Work out the finished part from the listing and answer in its coordinate system (mm). A direction names the side the tool comes from. Coordinates: 2 decimals unless noted, no trailing zeros. Order: outer loops, then holes, each group sorted by start corner. A loop starts at its lowest first (then second) coordinate and runs counter-clockwise, first axis right, second up. Notation, with made-up numbers: M -28.75,-7 L -11.75,-7 A28 cw -11.75,29 Z; hole C 61.5,34.5 d1. An arc over 180 degrees is marked long. Use a Markdown table: item, result.
from build123d import *

# Parameters (mm, degrees)
SKETCH1_W           = 88.9
SKETCH1_H           = 50.8
BOSS_EXTRUDE1_DEPTH = 12.7
SKETCH2_R           = 3.429
SKETCH2_R_2         = 2.286
CUT_EXTRUDE1_DEPTH  = 4.572
SKETCH3_R           = 2.286
CUT_EXTRUDE2_DEPTH  = 53.74706153
LPATTERN1_COUNT     = 2
LPATTERN1_PITCH     = 25.4
CUT_EXTRUDE3_DEPTH  = 69.685751798
SKETCH5_R           = 0.7874
CUT_EXTRUDE4_DEPTH  = 53.74706153
SKETCH6_R           = 2.286
CUT_EXTRUDE5_DEPTH  = 53.74706153


with BuildPart() as part:
    # Sketch1 → Boss-Extrude1 (new body)
    with BuildSketch(Plane(origin=(0, 0, 0), x_dir=(1, 0, 0), z_dir=(0, 1, 0))):
        Rectangle(SKETCH1_W, SKETCH1_H)
    extrude(amount=BOSS_EXTRUDE1_DEPTH)

    # Sketch2 → Cut-Extrude1 (cut)
    # profile 1 of 5: a face of its own
    with BuildSketch(Plane(origin=(0, 12.7, 0), x_dir=(1, 0, 0), z_dir=(0, 1, 0))):
        with Locations(Location((-34.29, 12.7, 0), (0, 0, 270))):
            Circle(SKETCH2_R)
        with Locations(Location((-34.29, 12.7, 0), (0, 0, 270))):
            Circle(SKETCH2_R_2, mode=Mode.SUBTRACT)
    # profile 2 of 5: a face of its own
    with BuildSketch(Plane(origin=(0, 12.7, 0), x_dir=(1, 0, 0), z_dir=(0, 1, 0))):
        with Locations(Location((-19.05, 12.7, 0), (0, 0, 270))):
            Circle(SKETCH2_R)
        with Locations(Location((-19.05, 12.7, 0), (0, 0, 270))):
            Circle(SKETCH2_R_2, mode=Mode.SUBTRACT)
    # profile 3 of 5: a face of its own
    with BuildSketch(Plane(origin=(0, 12.7, 0), x_dir=(1, 0, 0), z_dir=(0, 1, 0))):
        with Locations(Location((0, 12.7, 0), (0, 0, 270))):
            Circle(SKETCH2_R)
        with Locations(Location((0, 12.7, 0), (0, 0, 270))):
            Circle(SKETCH2_R_2, mode=Mode.SUBTRACT)
    # profile 4 of 5: a face of its own
    with BuildSketch(Plane(origin=(0, 12.7, 0), x_dir=(1, 0, 0), z_dir=(0, 1, 0))):
        with Locations(Location((19.05, 12.7, 0), (0, 0, 270))):
            Circle(SKETCH2_R)
        with Locations(Location((19.05, 12.7, 0), (0, 0, 270))):
            Circle(SKETCH2_R_2, mode=Mode.SUBTRACT)
    # profile 5 of 5: a face of its own
    with BuildSketch(Plane(origin=(0, 12.7, 0), x_dir=(1, 0, 0), z_dir=(0, 1, 0))):
        with Locations(Location((34.29, 12.7, 0), (0, 0, 270))):
            Circle(SKETCH2_R)
        with Locations(Location((34.29, 12.7, 0), (0, 0, 270))):
            Circle(SKETCH2_R_2, mode=Mode.SUBTRACT)
    cut_extrude1 = extrude(amount=-CUT_EXTRUDE1_DEPTH, mode=Mode.SUBTRACT)

    # Sketch3 → Cut-Extrude2 (cut, through all)
    with BuildSketch(Plane(origin=(0, 12.7, 0), x_dir=(1, 0, 0), z_dir=(0, 1, 0))):
        with Locations(Location((-34.29, 12.7, 0), (0, 0, 270))):
            Circle(SKETCH3_R)
        with Locations(Location((-19.05, 12.7, 0), (0, 0, 270))):
            Circle(SKETCH3_R)
        with Locations(Location((0, 12.7, 0), (0, 0, 270))):
            Circle(SKETCH3_R)
        with Locations(Location((19.05, 12.7, 0), (0, 0, 270))):
            Circle(SKETCH3_R)
        with Locations(Location((34.29, 12.7, 0), (0, 0, 270))):
            Circle(SKETCH3_R)
    extrude(amount=-CUT_EXTRUDE2_DEPTH, mode=Mode.SUBTRACT)

    # LPattern1: Cut-Extrude1 ×2
    with Locations(*[(0, 0, i * LPATTERN1_PITCH) for i in range(1, LPATTERN1_COUNT)]):
        add(cut_extrude1, mode=Mode.SUBTRACT)

    # Sketch4 → Cut-Extrude3 (cut, through all)
    with BuildSketch(Plane.XY.offset(25.4)):
        with BuildLine():
            Line((-28.702, 0), (-22.098, 0))
            ThreePointArc((-22.098, 0), (-25.4, 3.302), (-28.702, 0))
        make_face()
        with BuildLine():
            Line((-14.224, 0), (-4.572, 0))
            ThreePointArc((-4.572, 0), (-9.398, 4.826), (-14.224, 0))
        make_face()
        with BuildLine():
            Line((4.572, 0), (14.224, 0))
            ThreePointArc((14.224, 0), (9.398, 4.826), (4.572, 0))
        make_face()
        with BuildLine():
            Line((22.098, 0), (28.702, 0))
            ThreePointArc((28.702, 0), (25.4, 3.302), (22.098, 0))
        make_face()
    extrude(amount=-CUT_EXTRUDE3_DEPTH, mode=Mode.SUBTRACT)

    # Sketch5 → Cut-Extrude4 (cut, through all)
    with BuildSketch(Plane(origin=(0, 12.7, 0), x_dir=(1, 0, 0), z_dir=(0, 1, 0))):
        with Locations(Location((0, 0, 0), (0, 0, 270))):
            Circle(SKETCH5_R)
    extrude(amount=-CUT_EXTRUDE4_DEPTH, mode=Mode.SUBTRACT)

    # Sketch6 → Cut-Extrude5 (cut, through all)
    with BuildSketch(Plane(origin=(0, 12.7, 0), x_dir=(1, 0, 0), z_dir=(0, 1, 0))):
        with Locations(Location((-34.29, -12.7, 0), (0, 0, 270))):
            Circle(SKETCH6_R)
        with Locations(Location((-19.05, -12.7, 0), (0, 0, 270))):
            Circle(SKETCH6_R)
        with Locations(Location((0, -12.7, 0), (0, 0, 270))):
            Circle(SKETCH6_R)
        with Locations(Location((19.05, -12.7, 0), (0, 0, 270))):
            Circle(SKETCH6_R)
        with Locations(Location((34.29, -12.7, 0), (0, 0, 270))):
            Circle(SKETCH6_R)
    extrude(amount=-CUT_EXTRUDE5_DEPTH, mode=Mode.SUBTRACT)


solid = part.part
(1) Which of the six approach directions +Z, -Z, +X, -X, +Y, -Y give full straight-line access (tool end or side, diameter ignored) to faces 5 (the flat face through (-20, 8.128, -10)), 6 (the cylindrical face through (-20.441, 4.121, -14.514))?
Conclusion:
| item | result |
|---|---|
| face 5 | +Y |
| face 6 | +Y, -Y |
(2) A cutting plane is placed at A-A (x = -34.29). Determine the outline of the cut face in (y, z), then the cut area to 3 significant figures.
Conclusion:
| item | result |
|---|---|
| outline | M 0,-25.4 L 12.7,-25.4 L 12.7,-16.13 L 8.13,-16.13 L 8.13,-14.99 L 0,-14.99 Z; M 0,-10.41 L 8.13,-10.41 L 8.13,-9.27 L 12.7,-9.27 L 12.7,9.27 L 8.13,9.27 L 8.13,10.41 L 0,10.41 Z; M 0,14.99 L 8.13,14.99 L 8.13,16.13 L 12.7,16.13 L 12.7,25.4 L 0,25.4 Z |
| area | 508 mm2 |
(3) Straight lines are drawn through the part: L1, parallel to X at y = 10.7, z = 12.7; L2, parallel to Z at x = 1, y = 6; L3, parallel to X at y = 2, z = -10. For each, find the intervals that lie inside material, in ascending order.
Conclusion:
| item | result |
|---|---|
| L1 | -44.45 to -37.72, -30.86 to -22.48, -15.62 to -3.43, 3.43 to 15.62, 22.48 to 30.86, 37.72 to 44.45 |
| L2 | -25.4 to -14.76, -10.64 to 10.64, 14.76 to 25.4 |
| L3 | -44.45 to -28.03, -22.77 to -13.79, -5.01 to 5.01, 13.79 to 22.77, 28.03 to 44.45 |
(4) Given P1, Ø6, axis at x = -19.05, z = -12.7, coming from the +Y side; P2, Ø4, axis at x = -34.29, z = -12.7, coming from the -Y side, each flat-ended and moving along its own axis, determine where each tip first touches the part or whether it passes through.
Conclusion:
| item | result |
|---|---|
| P1 | y = 8.13 |
| P2 | through |
(5) A cutting plane is placed at B-B (y = 6.5). Give the number of separate pieces and of enclosed holes in the cut face, then the cut area to 3 significant figures.
Conclusion:
| item | result |
|---|---|
| separate pieces | 1 |
| enclosed holes | 11 |
| area | 4,350 mm2 |
(6) Determine the mould class of faces 1 (the flat face through (-1, 12.7, -6)), 2 (the flat face through (18, 8.128, -10)), 3 (the cylindrical face through (0.151, 10.446, 9.274)), 4 (the flat face through (-44.45, 6, 0)) for opening direction X: pulls with the +X half, pulls with the -X half, needs draft (parallel to the pull), parting line crosses it, or undercut.
Conclusion:
| item | result |
|---|---|
| face 1 | needs draft |
| face 2 | undercut |
| face 3 | undercut |
| face 4 | pulls with the -X half |
(7) A cutting plane is placed at C-C (z = -2). Determine the outline of the cut face in (x, y).
Conclusion:
| item | result |
|---|---|
| outline | M -44.45,0 L -28.7,0 A3.3 cw -22.1,0 L -14.22,0 A4.83 cw -4.57,0 L 4.57,0 A4.83 cw 14.22,0 L 22.1,0 A3.3 cw 28.7,0 L 44.45,0 L 44.45,12.7 L -44.45,12.7 Z |
